Drawing for the job (mm, zero at the part's lowest x, y, z). Give positions to 0.01 mm unless a question says otherwise; leave off trailing zeros. Order: outer loops, then holes, each group sorted by start corner. A loop starts at its lowest first (then second) coordinate and runs counter-clockwise, first axis right, second up. Notation, with made-up numbers: (-15.75, 77) - (7.25, 77) arc R8 cw to (7.25, 85) - close; hole circle Ø11 at (33, 88.5). An arc over 180 degrees is marked (long way). Use a Markdown table: item, result.
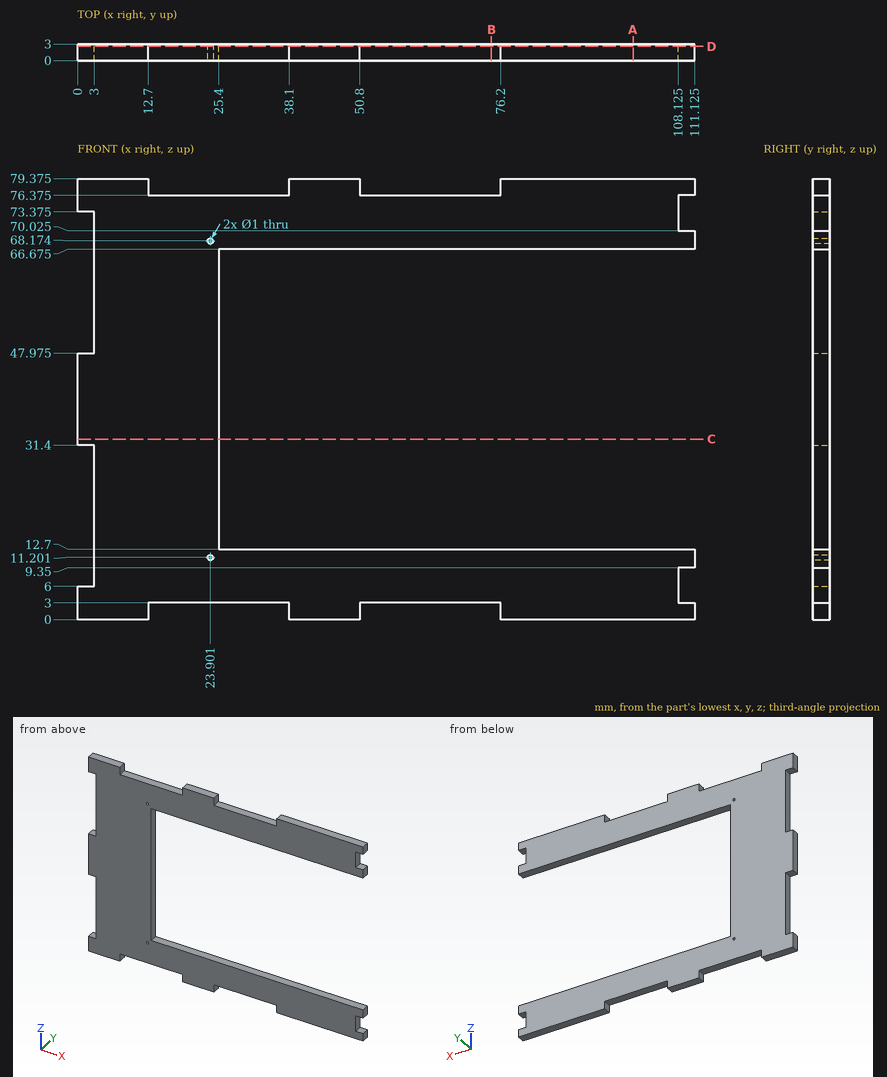
1) Slice it at A-A (x = 100). Write the cut outline in (y, z) (3 decimals).
Computed:
| item | result |
|---|---|
| outline | (0, 0) - (3, 0) - (3, 12.7) - (0, 12.7) - close; (0, 66.675) - (3, 66.675) - (3, 79.375) - (0, 79.375) - close |
2) Slice it at B-B (x = 74.5). Write the cut outline in (y, z) (3 decimals), and give its area (3 significant figures).
Computed:
| item | result |
|---|---|
| outline | (0, 3) - (3, 3) - (3, 12.7) - (0, 12.7) - close; (0, 66.675) - (3, 66.675) - (3, 76.375) - (0, 76.375) - close |
| area | 58.2 mm² |
3) Wall check: line 1 (Z direction, x = 68, y = 1.1) (3 decimals); line 2 (Z direction, x = 87.5, y = 1.15) (3 decimals); line 3 (X direction, y = 0.15, z = 76.5) (3 decimals). Give the ranges that are in metal, low to high. Write a range as from..to.
Computed:
| item | result |
|---|---|
| line 1 | z = 3..12.7, 66.675..76.375 |
| line 2 | z = 0..12.7, 66.675..79.375 |
| line 3 | x = 0..12.7, 38.1..50.8, 76.2..111.125 |
4) Pin check, flat tip, straight feed: P1, Ø1.5, axis at x = 14.5, y = 1, coming from the -Z side. Stop position of the tip, or through.
Computed:
| item | result |
|---|---|
| P1 | stops at z = 3 |
5) Slice it at C-C (z = 32.5). Write the cut outline in (x, y).
Computed:
| item | result |
|---|---|
| outline | (0, 0) - (25.4, 0) - (25.4, 3) - (0, 3) - close |
6) Slice it at D-D (y = 2.55). State how many separate pieces and enclosed holes the cut face has, and give its area (3 significant figures).
Computed:
| item | result |
|---|---|
| separate pieces | 1 |
| enclosed holes | 2 |
| area | 3,700 mm² |
